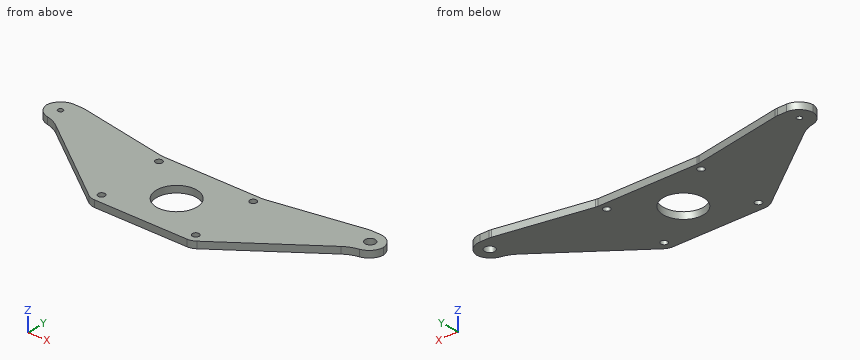
from build123d import *

# Parameters (mm, degrees)
EXTRUDE_1_DEPTH     = 4
FILLET_1_R          = 8
FILLET_2_R          = 20
SKETCH_3_R          = 2
CUT_EXTRUDE_2_DEPTH = 112.874930168
SKETCH_2_R          = 12
CUT_EXTRUDE_1_DEPTH = 112.874930168
SKETCH_4_R          = 1.5
CUT_EXTRUDE_3_DEPTH = 112.874930168
FILLET_3_R          = 9
SKETCH_5_R          = 3
SKETCH_5_R_2        = 1.5
CUT_EXTRUDE_4_DEPTH = 25


with BuildPart() as part:
    # 草图1 → 凸台-拉伸1 (new body)
    with BuildSketch(Plane.XY):
        Polygon((-100, 10), (-85, 10), (-30, 0), (30, 0), (85, 10), (100, 10), (100, -6), (90, -6), (30, -50), (-30, -50), (-90, -6), (-100, -6), align=None)
    extrude(amount=EXTRUDE_1_DEPTH)

    # 圆角1
    fillet_1_edges = [part.edges().sort_by_distance(p)[0] for p in [
        (-85, 10, 2),
        (-30, 0, 2),
        (30, 0, 2),
        (85, 10, 2),
        (30, -50, 2),
        (-30, -50, 2),
    ]]
    fillet(fillet_1_edges, radius=FILLET_1_R)

    # 圆角2
    fillet_2_edges = [part.edges().sort_by_distance(p)[0] for p in [
        (90, -6, 2),
        (-90, -6, 2),
    ]]
    fillet(fillet_2_edges, radius=FILLET_2_R)

    # 草图3 → 切除-拉伸2 (cut, through all)
    with BuildSketch(Plane(origin=(0, 0, 0), x_dir=(-1, 0, 0), z_dir=(0, 0, -1))):
        with Locations((-28, -4.5)):
            Circle(SKETCH_3_R)
        with Locations((-28, -44.5)):
            Circle(SKETCH_3_R)
    cut_extrude_2 = extrude(amount=-CUT_EXTRUDE_2_DEPTH, mode=Mode.SUBTRACT)

    # 草图2 → 切除-拉伸1 (cut, through all)
    with BuildSketch(Plane(origin=(0, 0, 0), x_dir=(-1, 0, 0), z_dir=(0, 0, -1))):
        with Locations((0, -25)):
            Circle(SKETCH_2_R)
    extrude(amount=-CUT_EXTRUDE_1_DEPTH, mode=Mode.SUBTRACT)

    # 镜向1: 切除-拉伸2 across plane
    add(cut_extrude_2.mirror(Plane(origin=(0, 0, 0), x_dir=(0, 0, 1), z_dir=(1, 0, 0))), mode=Mode.SUBTRACT)

    # 草图4 → 切除-拉伸3 (cut, through all)
    with BuildSketch(Plane(origin=(0, 0, 0), x_dir=(-1, 0, 0), z_dir=(0, 0, -1))):
        with Locations((92, 2)):
            Circle(SKETCH_4_R)
    cut_extrude_3 = extrude(amount=-CUT_EXTRUDE_3_DEPTH, mode=Mode.SUBTRACT)

    # 镜向2: 切除-拉伸3 across plane
    add(cut_extrude_3.mirror(Plane(origin=(0, 0, 0), x_dir=(0, 0, 1), z_dir=(1, 0, 0))), mode=Mode.SUBTRACT)

    # 圆角3
    # the kernel refuses this fillet: 9 mm, written as the material it takes off along each edge
    with BuildSketch(Plane(origin=(100, -6, -21.161183572), x_dir=(-0.9987150456948208, -0.05067797847972915, 0), z_dir=(0, 0, 1))) as fillet_3_piece_1:
        with BuildLine():
            CenterArc((8.559473009, -8.909698774), FILLET_3_R, 98.123197137, 78.971924263)
            Line((-0.428962402, -8.453596967), (-1.327805943, -8.407986787))
            Line((-1.327805943, -8.407986787), (-0.898843541, 0.045610181))
            Line((-0.898843541, 0.045610181), (0.045610181, 0.898843541))
            ThreePointArc((0.045610181, 0.898843541), (3.493764236, 0.723873235), (7.160582737, 0.890969877))
            Line((7.160582737, 0.890969877), (7.28775458, 0))
        make_face()
    extrude(amount=46.322367144, mode=Mode.SUBTRACT)
    with BuildSketch(Plane(origin=(100, 10, -22.5), x_dir=(0, -1, 0), z_dir=(0, 0, 1))) as fillet_3_piece_2:
        with BuildLine():
            CenterArc((FILLET_3_R, -FILLET_3_R), FILLET_3_R, 90, 90)
            Line((0, -FILLET_3_R), (0, 0))
            Line((0, 0), (FILLET_3_R, 0))
        make_face()
    extrude(amount=49, mode=Mode.SUBTRACT)
    with BuildSketch(Plane(origin=(-100, -6, -21.161183572), x_dir=(0.9987150456948208, -0.05067797847972878, 0), z_dir=(0, 0, 1))) as fillet_3_piece_3:
        with BuildLine():
            CenterArc((8.559473009, 8.909698774), FILLET_3_R, 182.9048786, 78.971924263)
            Line((-0.428962402, 8.453596967), (-1.327805943, 8.407986787))
            Line((-1.327805943, 8.407986787), (-0.898843541, -0.045610181))
            Line((-0.898843541, -0.045610181), (0.045610181, -0.898843541))
            ThreePointArc((0.045610181, -0.898843541), (3.493764236, -0.723873235), (7.160582737, -0.890969877))
            Line((7.160582737, -0.890969877), (7.28775458, 0))
        make_face()
    extrude(amount=46.322367144, mode=Mode.SUBTRACT)
    with BuildSketch(Plane(origin=(-100, 10, -22.5), x_dir=(0, -1, 0), z_dir=(0, 0, 1))) as fillet_3_piece_4:
        with BuildLine():
            CenterArc((FILLET_3_R, FILLET_3_R), FILLET_3_R, 180, 90)
            Line((0, FILLET_3_R), (0, 0))
            Line((0, 0), (FILLET_3_R, 0))
        make_face()
    extrude(amount=49, mode=Mode.SUBTRACT)

    # 草图5 → 切除-拉伸4 (cut)
    with BuildSketch(Plane(origin=(0, 0, 0), x_dir=(-1, 0, 0), z_dir=(0, 0, -1))):
        with Locations((-92, 2)):
            Circle(SKETCH_5_R)
        with Locations((-92, 2)):
            Circle(SKETCH_5_R_2, mode=Mode.SUBTRACT)
    extrude(amount=-CUT_EXTRUDE_4_DEPTH, mode=Mode.SUBTRACT)


solid = part.part
Here's how the part is built. I have some questions about the finished solid (model axes, mm). Give positions to 0.01 mm unless a question says otherwise; leave off trailing zeros. Order: outer loops, then holes, each group sorted by start corner. A loop starts at its lowest first (then second) coordinate and runs counter-clockwise, first axis right, second up. Notation, with made-up numbers: (-38, -33.5) -> (-30, -33.5) arc R28 ccw to (-30, -8.5) -> close; hole circle Ø8 at (-26, 64.5). An arc over 180 degrees is marked (long way). Use a Markdown table: item, result. Add a question column.
Item 1: Imagine slicing it at C-C on y = -19. Please give me the cut outline in (x, z).
Item 2: Will these pins go through, and if not, where does the flat tip stop? pin 1 (4 mm diameter, centred on x = -2.5, y = -34, fed in from +Z); pin 2 (1.2 mm diameter, centred on x = -0.5, z = 2.5, fed in from +Y); pin 3 (2 mm diameter, centred on y = -39, z = 0.5, fed in from -X).
Item 3: Imagine slicing it at A-A on x = 0. Please give me the cut outline in (y, z).
Item 4: Imagine slicing it at D-D on y = -4.5. Please give me the cut outline in (x, z), plus the area to 3 significant figures.
Item 5: I need wall thicknesses on line 1 (Y direction, x = 28, z = 2.6); line 2 (Y direction, x = 0, z = 1.8); line 3 (Y direction, x = -92, z = 2.3). Which ranges of each line are inside material? Lowest first, please.
Item 6: Imagine slicing it at B-B on z = 0.7. Please give me the cut outline in (x, y).
Data:
| question | item | result |
|---|---|---|
| 1 | outline | (-72.27, 0) -> (-10.39, 0) -> (-10.39, 4) -> (-72.27, 4) -> close; (10.39, 0) -> (72.27, 0) -> (72.27, 4) -> (10.39, 4) -> close |
| 2 | pin 1 | passes through |
| 2 | pin 2 | stops at y = 0 |
| 2 | pin 3 | stops at x = -46.36 |
| 3 | outline | (-50, 0) -> (-37, 0) -> (-37, 4) -> (-50, 4) -> close; (-13, 0) -> (0, 0) -> (0, 4) -> (-13, 4) -> close |
| 4 | outline | (-96.7, 0) -> (-30, 0) -> (-30, 4) -> (-96.7, 4) -> close; (-26, 0) -> (26, 0) -> (26, 4) -> (-26, 4) -> close; (30, 0) -> (96.7, 0) -> (96.7, 4) -> (30, 4) -> close |
| 4 | area | 742 mm² |
| 5 | line 1 | y = -49.98 to -46.5, -42.5 to -6.5, -2.5 to 0 |
| 5 | line 2 | y = -50 to -37, -13 to 0 |
| 5 | line 3 | y = -6.52 to 0.5, 3.5 to 9.94 |
| 6 | outline | (-99.97, 1.73) arc R9 ccw to (-92.72, -6.37) arc R20 cw to (-84.72, -9.87) -> (-32.11, -48.45) arc R8 ccw to (-27.38, -50) -> (27.38, -50) arc R8 ccw to (32.11, -48.45) -> (84.72, -9.87) arc R20 cw to (92.72, -6.37) arc R9 ccw to (99.97, 1.73) arc R9 ccw to (91, 10) -> (85.72, 10) arc R8 ccw to (84.29, 9.87) -> (30.71, 0.13) arc R8 cw to (29.28, 0) -> (-29.28, 0) arc R8 cw to (-30.71, 0.13) -> (-84.29, 9.87) arc R8 ccw to (-85.72, 10) -> (-91, 10) arc R9 ccw to start; hole circle Ø3 at (-92, 2); hole circle Ø4 at (-28, -44.5); hole circle Ø4 at (-28, -4.5); hole circle Ø24 at (0, -25); hole circle Ø4 at (28, -44.5); hole circle Ø4 at (28, -4.5); hole circle Ø6 at (92, 2) |
